```python
from build123d import *

# Parameters (mm, degrees)
SKETCH1_W           = 144
SKETCH1_H           = 50
BOSS_EXTRUDE1_DEPTH = 37.5
CUT_EXTRUDE1_DEPTH  = 75
SKETCH3_W           = 144
SKETCH3_H           = 51
CUT_EXTRUDE2_DEPTH  = 38
HOLE1_D             = 12


with BuildPart() as part:
    # Sketch1 → Boss-Extrude1 (new, symmetric)
    with BuildSketch(Plane.XY):
        Rectangle(SKETCH1_W, SKETCH1_H)
    extrude(amount=BOSS_EXTRUDE1_DEPTH, both=True)

    # Sketch2 → Cut-Extrude1 (cut)
    with BuildSketch(Plane.XY.offset(37.5)):
        with BuildLine():
            Line((-23.461355602, 25), (-72, 25))
            Line((-72, 25), (-72, -13))
            ThreePointArc((-72, -13), (-41.177929985, -2.37003937), (-23.461355602, 25))
        make_face()
        with BuildLine():
            Line((72, 25), (72, -13))
            ThreePointArc((72, -13), (41.177929985, -2.37003937), (23.461355602, 25))
            Line((23.461355602, 25), (72, 25))
        make_face()
    extrude(amount=-CUT_EXTRUDE1_DEPTH, mode=Mode.SUBTRACT)

    # Sketch3 → Cut-Extrude2 (cut)
    with BuildSketch(Plane(origin=(0, 25, 0), x_dir=(1, 0, 0), z_dir=(0, 1, 0))):
        Rectangle(SKETCH3_W, SKETCH3_H)
    extrude(amount=-CUT_EXTRUDE2_DEPTH, mode=Mode.SUBTRACT)

    # Hole1 (through all)
    with Locations(Plane.XY.offset(37.5)):
        with Locations((19, 0), (-19, 0)):
            Hole(HOLE1_D / 2)


solid = part.part
```
Source: CAD feature listing. Evaluate the final solid. Frame: model axes, mm. A direction names the side the tool comes from. Round coordinates to 2 decimals unless told otherwise and drop trailing zeros. Loops run counter-clockwise (first coordinate to the right, second up) from the corner with the lowest first, then second, coordinate; pieces in that order, holes last. Notation, with made-up numbers: M -18.5,-39 L 22.5,-39 A20 cw 22.5,-14 Z; hole C 60,22.5 d2. An arc over 180 degrees is marked long. Use a Markdown table: item, result. Add a question column.
1. Reachability of faces 1 (the flat face through (-1, -5, 37.5)), 2 (the flat face through (-1, -13, 0)) from +Z, -Z, +X, -X, +Y, -Y: full face, straight path, thin tool, end or side. Return the list, or none.
2. Section query A-A on x = 19. Return the cut outline in (y, z).
3. Line query: line 1 (Z direction, x = 24, y = -12.5); line 2 (X direction, y = -3, z = -33); line 3 (Y direction, x = -19, z = 28.25). Output: solid intervals per line, ascending.
4. Section query B-B on y = 2. Return the cut outline in (x, z).
5. Section query C-C on z = 30. Return the cut outline in (x, y), then the cut area to 3 significant figures.
6. Section query D-D on y = 22. Return the cut outline in (x, z), then the cut area to 3 significant figures.
7. Contact query for flat-ended pins moving along their axis: P1, Ø2, axis at x = 17, z = 4.5, coming from the +Y side; P2, Ø19, axis at x = 19, y = 0, coming from the +Z side. Output: stop coordinate, or through.
8. Mould query, pull axis X, two halves, no side actions, for faces 3 (the cylindrical face through (23.76, -3.65, 31.42)), 4 (the cylindrical face through (42, -3, -31)), 5 (the flat face through (-1, -5, -37.5)). Classes: pulls with the +X half, pulls with the -X half, needs draft (parallel to the pull), parting line crosses it, or undercut.
Reported:
| question | item | result |
|---|---|---|
| 1 | face 1 | +Z, +X, -X, +Y, -Y |
| 1 | face 2 | +X, -X, +Y |
| 2 | outline | M -25,-37.5 L -6,-37.5 L -6,-25.5 L -13,-25.5 L -13,25.5 L -6,25.5 L -6,37.5 L -25,37.5 Z; M 6,-37.5 L 25,-37.5 L 25,-25.5 L 6,-25.5 Z; M 6,25.5 L 25,25.5 L 25,37.5 L 6,37.5 Z |
| 3 | line 1 | z = -37.5 to -25.5, 25.5 to 37.5 |
| 3 | line 2 | x = -42 to -24.2, -13.8 to 13.8, 24.2 to 42 |
| 3 | line 3 | y = -25 to -6, 6 to 25 |
| 4 | outline | M -36.29,-37.5 L -24.66,-37.5 L -24.66,-25.5 L -36.29,-25.5 Z; M -36.29,25.5 L -24.66,25.5 L -24.66,37.5 L -36.29,37.5 Z; M -13.34,-37.5 L 13.34,-37.5 L 13.34,-25.5 L -13.34,-25.5 Z; M -13.34,25.5 L 13.34,25.5 L 13.34,37.5 L -13.34,37.5 Z; M 24.66,-37.5 L 36.29,-37.5 L 36.29,-25.5 L 24.66,-25.5 Z; M 24.66,25.5 L 36.29,25.5 L 36.29,37.5 L 24.66,37.5 Z |
| 5 | outline | M -72,-25 L 72,-25 L 72,-13 A50 cw 23.46,25 L -23.46,25 A50 cw -72,-13 Z; hole C -19,0 d12; hole C 19,0 d12 |
| 5 | area | 4,240 mm² |
| 6 | outline | M -24.3,-37.5 L 24.3,-37.5 L 24.3,-25.5 L -24.3,-25.5 Z; M -24.3,25.5 L 24.3,25.5 L 24.3,37.5 L -24.3,37.5 Z |
| 6 | area | 1,170 mm² |
| 7 | P1 | stops at y = -13 |
| 7 | P2 | stops at z = 37.5 |
| 8 | face 3 | undercut |
| 8 | face 4 | pulls with the +X half |
| 8 | face 5 | needs draft |
